Read the model definition and answer for the solid it produces. Units are mm, in the model's axes. Give positions to 0.01 mm unless a question says otherwise; leave off trailing zeros. Loops run counter-clockwise (first coordinate to the right, second up) from the corner with the lowest first, then second, coordinate; pieces in that order, holes last. Notation, with made-up numbers: (51.25, 8) - (86.25, 8) arc R33 cw to (86.25, 44) - close; hole circle Ø4 at (16.25, 37.25). An arc over 180 degrees is marked (long way). Write item = value, one per line.
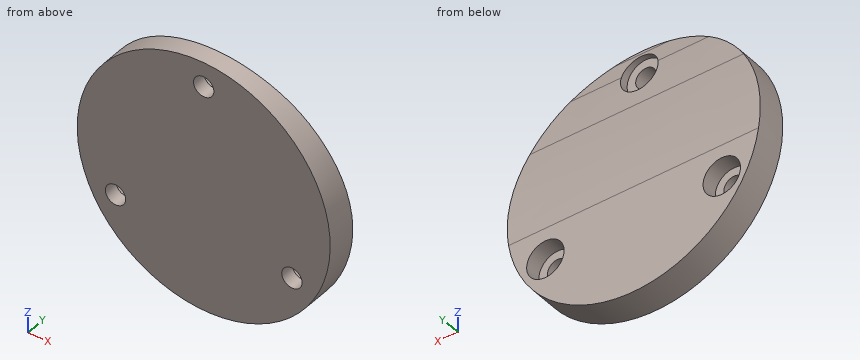
```python
from build123d import *

# Parameters (mm, degrees)
CROQUIS1_R              = 19.25
CROQUIS1_R_2            = 1.55
SALIENTE_EXTRUIR1_DEPTH = 4.6
CROQUIS2_R              = 2.85
CORTAR_EXTRUIR1_DEPTH   = 2.5
CORTAR_EXTRUIR2_START   = -20
CORTAR_EXTRUIR2_DEPTH   = 39.25


with BuildPart() as part:
    # Croquis1 → Saliente-Extruir1 (new body)
    with BuildSketch(Plane(origin=(0, 0, 0), x_dir=(1, 0, 0), z_dir=(0, 1, 0))):
        with Locations(Location((0, 0, 0), (0, 0, 270))):
            Circle(CROQUIS1_R)
        with Locations(Location((0, -15.5, 0), (0, 0, 270))):
            Circle(CROQUIS1_R_2, mode=Mode.SUBTRACT)
        with Locations(Location((13.423393759, 7.75, 0), (0, 0, 270))):
            Circle(CROQUIS1_R_2, mode=Mode.SUBTRACT)
        with Locations(Location((-13.423393759, 7.75, 0), (0, 0, 90))):
            Circle(CROQUIS1_R_2, mode=Mode.SUBTRACT)
    extrude(amount=SALIENTE_EXTRUIR1_DEPTH)

    # Croquis2 → Cortar-Extruir1 (cut)
    with BuildSketch(Plane(origin=(0, 4.6, 0), x_dir=(1, 0, 0), z_dir=(0, 1, 0))):
        with Locations(Location((-13.423393759, 7.75, 0), (0, 0, 270))):
            Circle(CROQUIS2_R)
        with Locations(Location((0, -15.5, 0), (0, 0, 270))):
            Circle(CROQUIS2_R)
        with Locations(Location((13.423393759, 7.75, 0), (0, 0, 270))):
            Circle(CROQUIS2_R)
    extrude(amount=-CORTAR_EXTRUIR1_DEPTH, mode=Mode.SUBTRACT)

    # Cortar-Extruir2: read off the stored shape, not the designer's step
    # Cortar-Extruir2 outline → Cortar-Extruir2 (cut)
    with BuildSketch(Plane(origin=(0, 0, 0), x_dir=(0, 0, -1), z_dir=(1, 0, 0)).offset(CORTAR_EXTRUIR2_START)):
        with BuildLine():
            add(Edge.make_bspline(
                [(2.936977636, 4.574175621), (1.790244303, 4.574175621), (0.64594889, 4.558108358), (-1.067035866, 4.512526979), (-1.637451159, 4.493737954), (-2.777118659, 4.449256149), (-3.347978215, 4.423479493), (-5.04815673, 4.33666012), (-6.144965171, 4.267295894), (-8.268827136, 4.110803555), (-9.295878077, 4.023634192), (-10.286640587, 3.929863966)],
                knots=[0, 0, 0, 0, 0.25, 0.25, 0.375, 0.375, 0.5, 0.5, 0.75, 0.75, 1, 1, 1, 1], degree=3))
            Line((2.936977636, 4.574175621), (19.25, 4.574175621))
            Line((19.25, 4.574175621), (20, 4.574175621))
            Line((20, 4.574175621), (20, 28.682505432))
            Line((20, 28.682505432), (9.143406809, 28.682505432))
            add(Edge.make_bspline(
                [(9.143406809, 28.682505432), (0.711546133, 17.325043273), (-7.611623296, 9.681788834), (-15.859834912, 4.6)],
                knots=[-1.666266403, -1.666266403, -1.666266403, -1.666266403, -0.863138153, -0.863138153, -0.863138153, -0.863138153], degree=3))
            add(Edge.make_bspline(
                [(-15.859834912, 4.6), (-16.832562085, 4.000695046), (-17.80424675, 3.437014777), (-18.774944235, 2.907068479)],
                knots=[-0.863138153, -0.863138153, -0.863138153, -0.863138153, -0.768423721, -0.768423721, -0.768423721, -0.768423721], degree=3))
            add(Edge.make_bspline(
                [(-16.107826284, 3.345164552), (-16.996272574, 3.2049165), (-17.885328598, 3.058510171), (-18.774944235, 2.907068479)],
                knots=[0.576630654, 0.576630654, 0.576630654, 0.576630654, 0.604116223, 0.604116223, 0.604116223, 0.604116223], degree=3))
            add(Edge.make_bspline(
                [(-10.286640587, 3.929863966), (-11.433287768, 3.821340113), (-12.490092354, 3.733147685), (-14.431499601, 3.557604756), (-15.316034761, 3.47015491), (-16.107826284, 3.345164552)],
                knots=[0, 0, 0, 0, 0.5, 0.5, 1, 1, 1, 1], degree=3))
        make_face()
        with BuildLine():
            add(Edge.make_bspline(
                [(-18.774944235, 2.907068479), (-18.933464547, 2.880083135), (-19.092002628, 2.85293791), (-19.250558194, 2.825639157)],
                knots=[0.604116223, 0.604116223, 0.604116223, 0.604116223, 0.609013868, 0.609013868, 0.609013868, 0.609013868], degree=3))
            add(Edge.make_bspline(
                [(-15.859834912, 4.6), (-16.832562085, 4.000695046), (-17.80424675, 3.437014777), (-18.774944235, 2.907068479)],
                knots=[-0.863138153, -0.863138153, -0.863138153, -0.863138153, -0.768423721, -0.768423721, -0.768423721, -0.768423721], degree=3))
            add(Edge.make_bspline(
                [(9.143406809, 28.682505432), (0.711546133, 17.325043273), (-7.611623296, 9.681788834), (-15.859834912, 4.6)],
                knots=[-1.666266403, -1.666266403, -1.666266403, -1.666266403, -0.863138153, -0.863138153, -0.863138153, -0.863138153], degree=3))
            Line((9.143406809, 28.682505432), (-19.854758161, 28.682505432))
            Line((-19.854758161, 28.682505432), (-19.854758161, 2.720897695))
            add(Edge.make_bspline(
                [(-19.250558194, 2.825639157), (-19.451930173, 2.790968638), (-19.653330356, 2.756050479), (-19.854758161, 2.720897695)],
                knots=[0.609013868, 0.609013868, 0.609013868, 0.609013868, 0.615234074, 0.615234074, 0.615234074, 0.615234074], degree=3))
        make_face()
    extrude(amount=CORTAR_EXTRUIR2_DEPTH, mode=Mode.SUBTRACT)


solid = part.part
```
1) Find the intervals of material crossed by probe 1 along X at (y, z) = (3.65, -7.75); probe 2 along Z at (x, y) = (3, 1.5); probe 3 along Y at (x, z) = (6, 3.5), in increasing order.
Output:
probe_1 = -17.62 to -16.27, -10.57 to 10.57, 16.27 to 17.62
probe_2 = -19.01 to 19.01
probe_3 = 0 to 4.42
2) Each of these flat-tipped pins is pushed along its axis until it touches: P1, Ø3, axis at x = -2, z = 2, coming from the +Y side; P2, Ø1.7, axis at x = -12, z = -7.5, coming from the +Y side; P3, Ø6.5, axis at x = 1, z = 14.5, coming from the +Y side. Where does it stop, or does it pass through?
Output:
P1 = 4.53
P2 = 2.1
P3 = 3.84
3) A cutting plane is placed at A-A on z = -7.75. Determine the outline of the cut face in (x, y), then the cut area to 3 significant figures.
Output:
outline = (-17.62, 0) - (-14.97, 0) - (-14.97, 2.1) - (-16.27, 2.1) - (-16.27, 4.57) - (-17.62, 4.57) - close; (-11.87, 0) - (11.87, 0) - (11.87, 2.1) - (10.57, 2.1) - (10.57, 4.57) - (-10.57, 4.57) - (-10.57, 2.1) - (-11.87, 2.1) - close; (14.97, 0) - (17.62, 0) - (17.62, 4.57) - (16.27, 4.57) - (16.27, 2.1) - (14.97, 2.1) - close
area = 120 mm²
4) A cutting plane is placed at B-B on y = 1.15. Determine the outline of the cut face in (x, z).
Output:
outline = circle Ø38.5 at (0, 0); hole circle Ø3.1 at (-13.42, -7.75); hole circle Ø3.1 at (0, 15.5); hole circle Ø3.1 at (13.42, -7.75)
5) A cutting plane is placed at C-C on z = -12. Determine the outline of the cut face in (x, y).
Output:
outline = (-15.05, 0) - (15.05, 0) - (15.05, 4.57) - (-15.05, 4.57) - close
